from build123d import *

# Parameters (mm, degrees)
SKETCH_19_W         = 15
SKETCH_19_H         = 110
EXTRUDE_11_DEPTH    = 16
SKETCH_23_R         = 19.628880498
CUT_EXTRUDE_4_DEPTH = 7.5
SKETCH_24_R         = 10
CUT_EXTRUDE_5_DEPTH = 27.5


with BuildPart() as part:
    # 草图19 → 旋转1 (revolve)
    with BuildSketch(Plane(origin=(0, 0, 0), x_dir=(0, 0, -1), z_dir=(1, 0, 0))):
        with Locations((-7.5, -55)):
            Rectangle(SKETCH_19_W, SKETCH_19_H)
    revolve(axis=Axis((0, 0, 0), (0, -1, 0)))

    # 草图22 → 凸台-拉伸11 (add, symmetric)
    with BuildSketch(Plane(origin=(0, 0, 0), x_dir=(0, 0, -1), z_dir=(1, 0, 0))):
        with BuildLine():
            Line((16, -110), (16, -160))
            ThreePointArc((16, -160), (0, -176), (-16, -160))
            Line((-16, -160), (-16, -110))
            ThreePointArc((-16, -110), (0, -94), (16, -110))
        make_face()
    extrude(amount=EXTRUDE_11_DEPTH, both=True)

    # 草图23 → 切除-拉伸4 (cut, symmetric)
    with BuildSketch(Plane(origin=(0, 0, 0), x_dir=(0, 0, -1), z_dir=(1, 0, 0))):
        with Locations((0, -160)):
            Circle(SKETCH_23_R)
    extrude(amount=CUT_EXTRUDE_4_DEPTH, both=True, mode=Mode.SUBTRACT)

    # 草图24 → 切除-拉伸5 (cut, symmetric)
    with BuildSketch(Plane(origin=(0, 0, 0), x_dir=(0, 0, -1), z_dir=(1, 0, 0))):
        with Locations((0, -160)):
            Circle(SKETCH_24_R)
    extrude(amount=CUT_EXTRUDE_5_DEPTH, both=True, mode=Mode.SUBTRACT)


solid = part.part
Build history of the part. All positions in model axes, mm. A direction names the side the tool comes from. Give positions to 0.01 mm unless a question says otherwise; leave off trailing zeros. Write each loop counter-clockwise with the first axis right and the second up, starting at its lowest first coordinate (ties: lowest second). Pieces come first, ordered by that corner, then holes. Notation, with made-up numbers: (9, 73.5) - (56, 73.5) arc R23 ccw to (56, 91.5) - close; hole circle Ø4 at (80.5, -12). An arc over 180 degrees is marked (long way). Use one line per item in the form item = value. Start each with the question number.
1. Band-saw the part on B-B on x = -12. Write the cut outline in (y, z), plus the area to 3 significant figures.
2. Probe line 1 (X direction, y = -145.5, z = -5.5); line 2 (Y direction, x = -9, z = 1); line 3 (Z direction, x = -11.5, y = -35). List the from-to ranges inside material, lowest first. Write a range as [from, to].
3. Drop flat-ended pins along their axis: pin 1 Ø1.5 at (x, y) = (-2, -102.5) entering from -Z; pin 2 Ø5 at (x, y) = (-9, -32) entering from -Z; pin 3 Ø12 at (y, z) = (-72, -12) entering from +X; pin 4 Ø1 at (x, z) = (8, -5.5) entering from +Y. Give the stop position or say it passes through.
4. Band-saw the part on A-A on z = 2.5. Write the cut outline in (x, y).
5. Band-saw the part on D-D on y = -32. Write the cut outline in (x, z).
6. 3-axis set-ups, long thin cutter, end or side, ignore diameter. For faces 1 (the face through (-7.5, -150, 4)), 2 (the face through (0, 0, 0)), 3 (the face through (7.34, -102.31, 14.03)): which of +Z, -Z, +X, -X, +Y, -Y reach the whole face in a straight line?
7. Band-saw the part on C-C on x = 0. Write the cut outline in (y, z), plus the area to 3 significant figures.
8. Two-plate mould, pull along X, no slides. Class faces 4 (the face through (7.5, -150, 4)), 5 (the face through (-0.66, -51.485, -14.985)), 6 (the face through (11.81, -169.76, 2.17)), 7 (the face through (0.105, -140.373, -0.262)): released by +X, released by -X, zero draft, split by the parting line, or undercut.
Conclusion:
q1.outline = (-160, -16) - (-110, -16) arc R16 ccw to (-96.77, -9) - (0, -9) - (0, 9) - (-96.77, 9) arc R16 ccw to (-110, 16) - (-160, 16) arc R16 ccw to start; hole circle Ø20 at (-160, 0)
q1.area = 3,800 mm²
q2.line_1 = [-16, -7.5], [7.5, 16]
q2.line_2 = [-175.97, -169.95], [-150.05, 0]
q2.line_3 = [-9.63, 9.63]
q3.pin_1 = -14.95
q3.pin_2 = -13.52
q3.pin_3 = 13.75
q3.pin_4 = 0
q4.outline = (-16, -175.8) - (-7.5, -175.8) - (-7.5, -169.68) - (-16, -169.68) - close; (-16, -150.32) - (-7.5, -150.32) - (-7.5, -140.53) - (7.5, -140.53) - (7.5, -150.32) - (16, -150.32) - (16, -94.2) - (14.79, -94.2) - (14.79, 0) - (-14.79, 0) - (-14.79, -94.2) - (-16, -94.2) - close; (7.5, -175.8) - (16, -175.8) - (16, -169.68) - (7.5, -169.68) - close
q5.outline = circle Ø30 at (0, 0)
q6.face_1 = -Y
q6.face_2 = +Z, -Z, +X, -X, +Y
q6.face_3 = +Y
q7.outline = (-148.63, -16) - (-110, -16) arc R16 ccw to (-104.43, -15) - (0, -15) - (0, 15) - (-104.43, 15) arc R16 ccw to (-110, 16) - (-148.63, 16) arc R19.63 cw to start
q7.area = 4,360 mm²
q8.face_4 = undercut
q8.face_5 = split by the parting line
q8.face_6 = zero draft
q8.face_7 = undercut
